Can you work these out from the model? Positions are in its coordinate system, mm. A direction names the side the tool comes from. Coordinates: 2 decimals unless noted, no trailing zeros. Order: outer loops, then holes, each group sorted by start corner. A loop starts at its lowest first (then second) coordinate and runs counter-clockwise, first axis right, second up. Notation, with made-up numbers: (65.5, 68) -> (116.5, 68) arc R20 ccw to (116.5, 93) -> close; hole circle Ø1 at (55.25, 33). An arc over 180 degrees is marked (long way). Return JSON: item names as keys, results as strings. Group by question number.
1) If we section it at A-A, the plane x = 17.5: Please give me the cut outline in (y, z).
2) For pin 1 (5 mm diameter, centred on x = -10.5, y = 9.5, fed in from +Z); pin 2 (1 mm diameter, centred on x = 8.5, z = 14, fed in from +Y); pin 3 (6.5 mm diameter, centred on x = -31.42, y = 15, fed in from -Z); pin 4 (7 mm diameter, centred on x = -7, y = 17.5, fed in from +Z), each with a flat end and sliding along its axis, tell me the tip position at first contact or that it passes through.
3) If I drill on probe 1 along Y at (x, z) = (32.5, 2.25); probe 2 along Y at (x, z) = (6.5, 14.25); probe 3 along Z at (x, y) = (40, -22), over which ranges is the centre line in solid material (lowest first)? Write a range as from..to.
4) If we section it at C-C, the plane y = -28: State how many separate pieces and enclosed holes the cut face has, then the cut area to 3 significant figures.
5) If we section it at D-D, the plane z = 11: Please give me the cut outline in (x, y) (1 decimal), then the cut area to 3 significant figures.
6) If we section it at B-B, the plane z = 3.75: Please give me the cut outline in (x, y) (1 decimal), then the cut area to 3 significant figures.
7) For faces 4 (the flat face through (5, -6, 23)), 5 (the flat face through (3, -27, 6.5)), which set-ups out of +Z, -Z, +X, -X, +Y, -Y let a thin tool reach every point of the face, with its end or its side?
8) Thinking about a two-plate mould opening in Y: for faces 1 (the cylindrical face through (30.06, 13.3, 4)), 2 (the flat face through (3, 15, 6.5)), 3 (the flat face through (3, -19.9, 15)), which applies, +Y half, -Y half, draft (parallel to the pull), parting line (faces both ways), or undercut?
from build123d import *

# Parameters (mm, degrees)
F0_R         = 2.8
F1_DEPTH     = 6.5
F3_DEPTH     = 16.5
F4_T1_DEPTH  = 63.8184719387
F4_T3_DEPTH  = 45.8
F4_T5_DEPTH  = 9
F4_T7_DEPTH  = 9
F4_T10_ANGLE = 90
F4_T12_ANGLE = 120.4504110916
F4_T14_ANGLE = 90
F4_T16_ANGLE = 90
F4_T18_ANGLE = 29.7747944542
F4_T20_ANGLE = 29.7747944542
F4_T22_ANGLE = 29.7747944542
F4_T26_ANGLE = 35.5690080159
F4_T29_ANGLE = 90
F4_T33_ANGLE = 35.5690080159
F4_T36_ANGLE = 29.7747944542
F5_SIZE      = 1.56


# Not quite as in the source:
# - a fillet or chamfer that OpenCascade refuses, or shapes differently, is made with other operations: its cross-section is extruded or revolved along the edge and cut away or added


with BuildPart() as f1:
    # F0 (on Top) → F1 (new body)
    with BuildSketch(Plane.XY):
        with BuildLine():
            Line((-38.8770699501, 16.9000072956), (-38.8770699501, -28.8999927044))
            ThreePointArc((-38.8770699501, -28.8999927044), (-37.412603856, -32.4355266103), (-33.8770699501, -33.8999927044))
            Line((-33.8770699501, -33.8999927044), (29.9414019886, -33.8999927044))
            ThreePointArc((29.9414019886, -33.8999927044), (32.5106042183, -33.5643188528), (34.9073236464, -32.579832685))
            ThreePointArc((34.9073236464, -32.579832685), (50.3229300499, -5.9999927044), (34.9073236464, 20.5798472762))
            ThreePointArc((34.9073236464, 20.5798472762), (32.5106042183, 21.564333444), (29.9414019886, 21.9000072956))
            Line((29.9414019886, 21.9000072956), (-33.8770699501, 21.9000072956))
            ThreePointArc((-33.8770699501, 21.9000072956), (-37.412603856, 20.4355412015), (-38.8770699501, 16.9000072956))
        make_face()
        with Locations((-31.4170904458, -26.9999932498)):
            Circle(F0_R, mode=Mode.SUBTRACT)
        with Locations((32.2829300499, -26.9999927044)):
            Circle(F0_R, mode=Mode.SUBTRACT)
        with Locations((-31.4170904458, 15.0000071153)):
            Circle(F0_R, mode=Mode.SUBTRACT)
        with Locations((32.2829300499, 15.0000072956)):
            Circle(F0_R, mode=Mode.SUBTRACT)
    extrude(amount=F1_DEPTH)

    # F2 (on face) → F3 (join)
    with BuildSketch(Plane.XY.offset(6.5)):
        with BuildLine():
            Line((-38.8770699501, 7.9000072956), (-38.8770699501, -5.9999927044))
            Line((-38.8770699501, -5.9999927044), (-38.8770699501, -19.8999927044))
            Line((-38.8770699501, -19.8999927044), (46.9864613892, -19.8999927044))
            ThreePointArc((46.9864613892, -19.8999927044), (50.3229300499, -5.9999927044), (46.9864613892, 7.9000072956))
            Line((46.9864613892, 7.9000072956), (-38.8770699501, 7.9000072956))
        make_face()
    extrude(amount=F3_DEPTH)

    # F4: fillet of radius 0.5 on 18 edges, made by hand

    # F4_s2 → F4_t1 (cut)
    with BuildSketch(Plane.YZ.offset(-33.8770699501)):
        with BuildLine():
            ThreePointArc((21.9000072956, 0.5), (21.7535606862, 0.1464466094), (21.4000072956, 0))
            Line((21.4000072956, 0), (21.9000072956, 0))
            Line((21.9000072956, 0), (21.9000072956, 0.5))
        make_face()
        with BuildLine():
            ThreePointArc((21.9000072956, 6), (21.7535606862, 6.3535533906), (21.4000072956, 6.5))
            Line((21.4000072956, 6.5), (21.9000072956, 6.5))
            Line((21.9000072956, 6.5), (21.9000072956, 6))
        make_face()
        with BuildLine():
            ThreePointArc((-33.3999927044, 6.5), (-33.753546095, 6.3535533906), (-33.8999927044, 6))
            Line((-33.8999927044, 6), (-33.8999927044, 6.5))
            Line((-33.8999927044, 6.5), (-33.3999927044, 6.5))
        make_face()
        with BuildLine():
            ThreePointArc((-33.3999927044, 0), (-33.753546095, 0.1464466094), (-33.8999927044, 0.5))
            Line((-33.8999927044, 0.5), (-33.8999927044, 0))
            Line((-33.8999927044, 0), (-33.3999927044, 0))
        make_face()
    extrude(amount=F4_T1_DEPTH, mode=Mode.SUBTRACT)

    # F4_s4 → F4_t3 (cut)
    with BuildSketch(Plane.XZ.offset(-16.9000072956)):
        with BuildLine():
            ThreePointArc((-38.8770699501, 0.5), (-38.7306233407, 0.1464466094), (-38.3770699501, 0))
            Line((-38.3770699501, 0), (-38.8770699501, 0))
            Line((-38.8770699501, 0), (-38.8770699501, 0.5))
        make_face()
    extrude(amount=F4_T3_DEPTH, mode=Mode.SUBTRACT)

    # F4_s6 → F4_t5 (cut)
    with BuildSketch(Plane.XZ.offset(-16.9000072956)):
        with BuildLine():
            ThreePointArc((-38.8770699501, 6), (-38.7306233407, 6.3535533906), (-38.3770699501, 6.5))
            Line((-38.3770699501, 6.5), (-38.8770699501, 6.5))
            Line((-38.8770699501, 6.5), (-38.8770699501, 6))
        make_face()
    extrude(amount=F4_T5_DEPTH, mode=Mode.SUBTRACT)

    # F4_s8 → F4_t7 (cut)
    with BuildSketch(Plane.XZ.offset(19.8999927044)):
        with BuildLine():
            ThreePointArc((-38.8770699501, 6), (-38.7306233407, 6.3535533906), (-38.3770699501, 6.5))
            Line((-38.3770699501, 6.5), (-38.8770699501, 6.5))
            Line((-38.8770699501, 6.5), (-38.8770699501, 6))
        make_face()
    extrude(amount=F4_T7_DEPTH, mode=Mode.SUBTRACT)

    # F4_s9 → F4_t10 (revolve, cut)
    with BuildSketch(Plane.YZ.offset(-33.8770699501)):
        with BuildLine():
            ThreePointArc((21.9000072956, 0.5), (21.7535606862, 0.1464466094), (21.4000072956, 0))
            Line((21.4000072956, 0), (21.9000072956, 0))
            Line((21.9000072956, 0), (21.9000072956, 0.5))
        make_face()
    revolve(axis=Axis((-33.8770699501, 16.9000072956, 0), (0, 0, 1)), revolution_arc=F4_T10_ANGLE, mode=Mode.SUBTRACT)

    # F4_s11 → F4_t12 (revolve, cut)
    with BuildSketch(Plane(origin=(12.2560283734, 7.0119353437, 0), x_dir=(0, 0, 1), z_dir=(-0.8679839981, -0.4965921658, 0))):
        with BuildLine():
            ThreePointArc((0, -45.1134768811), (0.1464466094, -45.4670302717), (0.5, -45.6134768811))
            Line((0.5, -45.6134768811), (0, -45.6134768811))
            Line((0, -45.6134768811), (0, -45.1134768811))
        make_face()
    revolve(axis=Axis((19.7004300499, -5.9999927044, 0), (0, 0, 1)), revolution_arc=F4_T12_ANGLE, mode=Mode.SUBTRACT)

    # F4_s13 → F4_t14 (revolve, cut)
    with BuildSketch(Plane.YZ.offset(-33.8770699501)):
        with BuildLine():
            ThreePointArc((21.9000072956, 6), (21.7535606862, 6.3535533906), (21.4000072956, 6.5))
            Line((21.4000072956, 6.5), (21.9000072956, 6.5))
            Line((21.9000072956, 6.5), (21.9000072956, 6))
        make_face()
    revolve(axis=Axis((-33.8770699501, 16.9000072956, 6.5), (0, 0, 1)), revolution_arc=F4_T14_ANGLE, mode=Mode.SUBTRACT)

    # F4_s15 → F4_t16 (revolve, cut)
    with BuildSketch(Plane.XZ.offset(28.8999927044)):
        with BuildLine():
            ThreePointArc((-38.3770699501, 0), (-38.7306233407, 0.1464466094), (-38.8770699501, 0.5))
            Line((-38.8770699501, 0.5), (-38.8770699501, 0))
            Line((-38.8770699501, 0), (-38.3770699501, 0))
        make_face()
    revolve(axis=Axis((-33.8770699501, -28.8999927044, 0), (0, 0, 1)), revolution_arc=F4_T16_ANGLE, mode=Mode.SUBTRACT)

    # F4_s17 → F4_t18 (revolve, cut)
    with BuildSketch(Plane.YZ.offset(29.9414019886)):
        with BuildLine():
            ThreePointArc((-33.3999927044, 0), (-33.753546095, 0.1464466094), (-33.8999927044, 0.5))
            Line((-33.8999927044, 0.5), (-33.8999927044, 0))
            Line((-33.8999927044, 0), (-33.3999927044, 0))
        make_face()
    revolve(axis=Axis((29.9414019886, -23.8999927044, 0), (0, 0, 1)), revolution_arc=F4_T18_ANGLE, mode=Mode.SUBTRACT)

    # F4_s19 → F4_t20 (revolve, cut)
    with BuildSketch(Plane(origin=(17.4284307256, -9.9711770948, 0), x_dir=(0, 0, 1), z_dir=(0.8679839981, -0.4965921658, 0))):
        with BuildLine():
            ThreePointArc((0, -34.6976815693), (0.1464466094, -35.0512349599), (0.5, -35.1976815693))
            Line((0.5, -35.1976815693), (0, -35.1976815693))
            Line((0, -35.1976815693), (0, -34.6976815693))
        make_face()
    revolve(axis=Axis((29.9414019886, 11.9000072956, 0), (0, 0, 1)), revolution_arc=F4_T20_ANGLE, mode=Mode.SUBTRACT)

    # F4_s21 → F4_t22 (revolve, cut)
    with BuildSketch(Plane(origin=(17.4284307256, -9.9711770948, 0), x_dir=(0, 0, 1), z_dir=(0.8679839981, -0.4965921658, 0))):
        with BuildLine():
            ThreePointArc((6.5, -34.6976815693), (6.3535533906, -35.0512349599), (6, -35.1976815693))
            Line((6, -35.1976815693), (6.5, -35.1976815693))
            Line((6.5, -35.1976815693), (6.5, -34.6976815693))
        make_face()
    revolve(axis=Axis((29.9414019886, 11.9000072956, 6.5), (0, 0, 1)), revolution_arc=F4_T22_ANGLE, mode=Mode.SUBTRACT)


with BuildPart() as f4_tool24:
    # F4_s25 → F4_t26 (revolve)
    with BuildSketch(Plane(origin=(5.7033446243, -12.4249727464, 0), x_dir=(0, 0, 1), z_dir=(0.4171723997, -0.9088273703, 0))):
        with BuildLine():
            ThreePointArc((6.5, -45.5237586807), (6.3535533906, -45.8773120713), (6, -46.0237586807))
            Line((6, -46.0237586807), (6.5, -46.0237586807))
            Line((6.5, -46.0237586807), (6.5, -45.5237586807))
        make_face()
    revolve(axis=Axis((19.7004300499, -5.9999927044, 6.5), (0, 0, 1)), revolution_arc=F4_T26_ANGLE)

    split(bisect_by=Plane.XZ.offset(-7.9000072956), keep=Keep.BOTTOM)


with BuildPart() as f1_1:
    add(f1.part)

    # F4_t23: cut F4_tool24
    add(f4_tool24.part, mode=Mode.SUBTRACT)

    # F4_s28 → F4_t29 (revolve, cut)
    with BuildSketch(Plane.XZ.offset(28.8999927044)):
        with BuildLine():
            ThreePointArc((-38.8770699501, 6), (-38.7306233407, 6.3535533906), (-38.3770699501, 6.5))
            Line((-38.3770699501, 6.5), (-38.8770699501, 6.5))
            Line((-38.8770699501, 6.5), (-38.8770699501, 6))
        make_face()
    revolve(axis=Axis((-33.8770699501, -28.8999927044, 6.5), (0, 0, 1)), revolution_arc=F4_T29_ANGLE, mode=Mode.SUBTRACT)


with BuildPart() as f4_tool31:
    # F4_s32 → F4_t33 (revolve)
    with BuildSketch(Plane(origin=(12.2560283734, 7.0119353437, 0), x_dir=(0, 0, 1), z_dir=(-0.8679839981, -0.4965921658, 0))):
        with BuildLine():
            ThreePointArc((6.5, -45.1134768811), (6.3535533906, -45.4670302717), (6, -45.6134768811))
            Line((6, -45.6134768811), (6.5, -45.6134768811))
            Line((6.5, -45.6134768811), (6.5, -45.1134768811))
        make_face()
    revolve(axis=Axis((19.7004300499, -5.9999927044, 6.5), (0, 0, 1)), revolution_arc=F4_T33_ANGLE)

    split(bisect_by=Plane.XZ.offset(19.8999927044), keep=Keep.TOP)


with BuildPart() as f1_2:
    add(f1_1.part)

    # F4_t30: cut F4_tool31
    add(f4_tool31.part, mode=Mode.SUBTRACT)

    # F4_s35 → F4_t36 (revolve, cut)
    with BuildSketch(Plane.YZ.offset(29.9414019886)):
        with BuildLine():
            ThreePointArc((-33.3999927044, 6.5), (-33.753546095, 6.3535533906), (-33.8999927044, 6))
            Line((-33.8999927044, 6), (-33.8999927044, 6.5))
            Line((-33.8999927044, 6.5), (-33.3999927044, 6.5))
        make_face()
    revolve(axis=Axis((29.9414019886, -23.8999927044, 6.5), (0, 0, 1)), revolution_arc=F4_T36_ANGLE, mode=Mode.SUBTRACT)

    # F5
    f5_edges = [f1_2.edges().sort_by_distance(p)[0] for p in [
        (-34.21709, 15.000007, 0),
        (-34.21709, -26.999993, 0),
        (29.48293, -26.999993, 0),
        (29.48293, 15.000007, 0),
    ]]
    chamfer(f5_edges, length=F5_SIZE)


solid = f1_2.part
Result sheet:
{
 "1": {"outline": "(-33.9, 0.5) arc R0.5 ccw to (-33.4, 0) -> (21.4, 0) arc R0.5 ccw to (21.9, 0.5) -> (21.9, 6) arc R0.5 ccw to (21.4, 6.5) -> (7.9, 6.5) -> (7.9, 23) -> (-19.9, 23) -> (-19.9, 6.5) -> (-33.4, 6.5) arc R0.5 ccw to (-33.9, 6) -> close"},
 "2": {"pin 1": "stops at z = 23", "pin 2": "stops at y = 7.9", "pin 3": "stops at z = 1.11", "pin 4": "stops at z = 6.5"},
 "3": {"probe 1": "y = -33.57..-29.79, -24.21..12.21, 17.79..21.57", "probe 2": "y = -19.9..7.9", "probe 3": "z = 0..6.5"},
 "4": {"separate pieces": "3", "enclosed holes": "0", "area": "446 mm2"},
 "5": {"outline": "(-38.9, -19.9) -> (47, -19.9) arc R30.6 ccw to (47, 7.9) -> (-38.9, 7.9) -> close", "area": "2,450 mm2"},
 "6": {"outline": "(-38.9, -28.9) arc R5 ccw to (-33.9, -33.9) -> (29.9, -33.9) arc R10 ccw to (34.9, -32.6) arc R30.6 ccw to (34.9, 20.6) arc R10 ccw to (29.9, 21.9) -> (-33.9, 21.9) arc R5 ccw to (-38.9, 16.9) -> close; hole circle Ø5.6 at (-31.4, -27); hole circle Ø5.6 at (-31.4, 15); hole circle Ø5.6 at (32.3, -27); hole circle Ø5.6 at (32.3, 15)", "area": "4,590 mm2"},
 "7": {"face 4": "+Z, +X, -X, +Y, -Y", "face 5": "+Z, +X, -X, -Y"},
 "8": {"face 1": "undercut", "face 2": "draft", "face 3": "-Y half"}
}
